Geometry check sheet. Reference: drawing and pictorial views, mm from the part's lowest x, y, z. Give positions to 0.01 mm unless a question says otherwise; leave off trailing zeros. Order: outer loops, then holes, each group sorted by start corner. A loop starts at its lowest first (then second) coordinate and runs counter-clockwise, first axis right, second up. Notation, with made-up numbers: (65.5, 63.25) -> (90.5, 63.25) arc R22 ccw to (90.5, 90.25) -> close; hole circle Ø2 at (-14, -3). An arc over 180 degrees is marked (long way). Write each question's results on one line, items separated by ' | '.
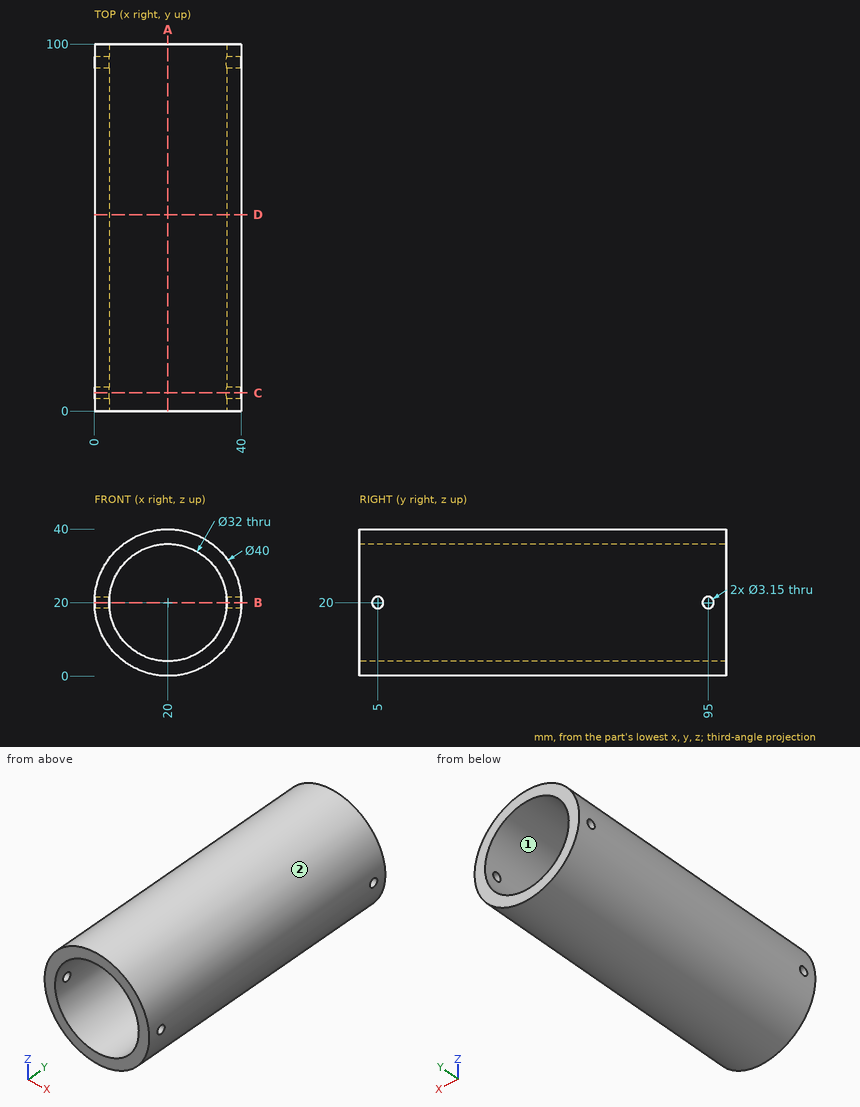
1. Section check A-A on x = 20. Record the cut outline in (y, z).
Verdict:
outline: (0, 0) -> (100, 0) -> (100, 4) -> (0, 4) -> close; (0, 36) -> (100, 36) -> (100, 40) -> (0, 40) -> close
2. Material ranges on probe 1 along Y at (x, z) = (38.7, 20) (3 decimals); probe 2 along X at (y, z) = (43.5, 30.5); probe 3 along Z at (x, y) = (33, 73.5), recorded low to high. Write a range as from..to.
Verdict:
probe 1: y = 0..3.425, 6.575..93.425, 96.575..100 | probe 2: x = 2.98..7.93, 32.07..37.02 | probe 3: z = 4.8..10.67, 29.33..35.2
3. Section check C-C on y = 5. Record the cut outline in (x, z) (3 decimals).
Verdict:
outline: (0.062, 18.425) arc R20 ccw to (39.938, 18.425) -> (35.922, 18.425) arc R16 cw to (4.078, 18.425) -> close; (0.062, 21.575) -> (4.078, 21.575) arc R16 cw to (35.922, 21.575) -> (39.938, 21.575) arc R20 ccw to start
4. Mould release check, pull along Z, two halves, no side actions. Record for the marked faces 1 and 2: +Z half, -Z half, draft (parallel to the pull), parting line (faces both ways), or undercut.
Verdict:
face 1: undercut | face 2: parting line
5. Section check B-B on z = 20. Record the cut outline in (x, y) (3 decimals), then the cut area to 3 significant figures.
Verdict:
outline: (0, 0) -> (4, 0) -> (4, 3.425) -> (0, 3.425) -> close; (0, 6.575) -> (4, 6.575) -> (4, 93.425) -> (0, 93.425) -> close; (0, 96.575) -> (4, 96.575) -> (4, 100) -> (0, 100) -> close; (36, 0) -> (40, 0) -> (40, 3.425) -> (36, 3.425) -> close; (36, 6.575) -> (40, 6.575) -> (40, 93.425) -> (36, 93.425) -> close; (36, 96.575) -> (40, 96.575) -> (40, 100) -> (36, 100) -> close | area: 750 mm^2
6. Gauge pin test, flat ends, axial feed: pin 1 Ø1 at (x, y) = (26, 36) entering from +Z; pin 2 Ø8 at (x, z) = (30.5, 30.5) entering from +Y; pin 3 Ø8 at (y, z) = (55.5, 24.5) entering from +X; pin 4 Ø4 at (x, y) = (23.5, 30.5) entering from -Z. Record the tip position at first contact, or that the pin passes through.
Verdict:
pin 1: stops at z = 39.23 | pin 2: stops at y = 100 | pin 3: stops at x = 39.99 | pin 4: stops at z = 0.06
7. Section check D-D on y = 53.5. Record the cut outline in (x, z), then the cut area to 3 significant figures.
Verdict:
outline: circle Ø40 at (20, 20); hole circle Ø32 at (20, 20) | area: 452 mm^2
